Here's how the part is built. I have some questions about the finished solid (model axes, mm). A direction names the side the tool comes from. Give positions to 0.01 mm unless a question says otherwise; leave off trailing zeros. Write each loop counter-clockwise with the first axis right and the second up, starting at its lowest first coordinate (ties: lowest second). Pieces come first, ordered by that corner, then holes. Notation, with made-up numbers: (44.5, 86.25) -> (70.5, 86.25) arc R20 ccw to (70.5, 107.25) -> close; hole circle Ø3 at (73, 4.5). An arc over 180 degrees is marked (long way). Put each result on its own line as item: value. Start each with the question number.
Autodesk Inventor part; units mm, degrees
ref_plane "YZ Plane" through (0, 0, 0) normal (1, 0, 0) x (0, 1, 0)
ref_plane "XZ Plane" through (0, 0, 0) normal (0, 1, 0) x (-1, 0, 0)
ref_plane "XY Plane" through (0, 0, 0) normal (0, 0, 1) x (1, 0, 0)
sketch "Szkic1" plane through (0, 0, 0) normal (1, 0, 0) x (0, 1, 0)
  line L0 (13, 21) -> (0, 21)
  line L1 (0, 21) -> (0, -21)
  line L2 (0, -21) -> (13, -21)
  line L3 (13, -21) -> (13, 21)
  line L4 (0, 0) -> (13, 0) construction
  dimension "d0" = 42
  dimension "d1" = 13
extrude "Wyciągnięcie proste3" add sketch "Szkic1" along normal blind 16
chamfer "Faza1" distance 4 angle 45 2 edges at (8, 0, 21) (8, 0, -21)
sketch "Szkic6" plane through (0, 0, -17) normal (0, -1, 0) x (1, 0, 0)
  line L0 (0, -4) -> (16, -4)
  line L1 (0, 34) -> (0, 0)
  line L2 (16, 34) -> (16, 0)
  point P0 (0, 17)
  point P1 (10, 11)
  dimension "d28" = 15
  dimension "d53" = 6
hole "Otwór2" at (10, 0, -6) direction (0, 1, 0) diameter 3 end through all
sketch "Szkic7" plane through (0, 0, -17) normal (0, -1, 0) x (1, 0, 0)
  line L0 (16, 38) -> (0, 38)
  circle A0 centre (10, 11) radius 1.5
  point P0 (0, 17)
  point P1 (10, 28.5)
  dimension "d37" = 9.5
hole "Otwór3" at (10, 0, 11.5) direction (0, 1, 0) diameter 4 end through all
thread "Gwint2"
sketch "Szkic8" plane through (0, 0, 0) normal (-1, 0, 0) x (0, 0, 1)
  line L0 (21, 13) -> (-17, 13)
  line L1 (-17, 13) -> (-17, 9)
  line L2 (-12, 4) -> (21, 4)
  line L3 (21, 4) -> (21, 13)
  line L4 (17, 0) -> (-17, 0)
  line L5 (-21, 4) -> (-21, 13)
  line L6 (-12, 4) -> (-17, 9)
  point P0 (0, 0)
  point P1 (-17, 4)
  dimension "d55" = 4
  dimension "d56" = 4
  dimension "d59" = 5
  dimension "d60" = 5
extrude "Wyciągnięcie proste5" cut sketch "Szkic8" against normal blind 3
sketch "Szkic9" plane through (16, 0, 0) normal (1, 0, 0) x (0, 0, -1)
  line L0 (-17, 0) -> (17, 0)
  line L1 (21, 4) -> (21, 13)
  point P0 (0, 0)
  point P1 (16.5, 4.5)
  dimension "d63" = 4.5
  dimension "d64" = 4.5
hole "Otwór4" at (16, 4.5, -16.5) direction (-1, 0, 0) diameter 3 end through all
thread "Gwint5"
sketch "Szkic10" plane through (16, 0, 0) normal (1, 0, 0) x (0, 0, -1)
  line L0 (21, 13) -> (-21, 13)
  line L1 (21, 13) -> (9, 13)
  line L2 (9, 13) -> (9, 26)
  line L3 (9, 26) -> (21, 26)
  line L4 (21, 26) -> (21, 13)
  point P0 (0, 0)
  dimension "d74" = 12
  dimension "d75" = 13
extrude "Wyciągnięcie proste6" add sketch "Szkic10" against normal up to surface (16 mm away)
sketch "Szkic11" plane through (0, 0, 0) normal (-1, 0, 0) x (0, 0, 1)
  line L0 (-17, 9) -> (-17, 13)
  line L1 (-9, 26) -> (-21, 26)
  line L2 (-17, 13) -> (-9, 13)
  line L3 (-9, 13) -> (-9, 26)
  line L4 (-9, 26) -> (-17, 26)
  line L5 (-17, 26) -> (-17, 13)
  point P0 (0, 0)
extrude "Wyciągnięcie proste7" cut sketch "Szkic11" against normal up to surface (3 mm away)
fillet "Zaokrąglenie2" radius 2 1 edges at (9.5, 13, -9)
sketch "Szkic12" plane through (16, 0, 0) normal (1, 0, 0) x (0, 0, -1)
  circle A0 centre (16.5, 4.5) radius 1.5
  circle A1 centre (16.5, 4.5) radius 2.75
  point P0 (0, 0)
  dimension "d83" = 1.25
extrude "Wyciągnięcie proste8" cut sketch "Szkic12" against normal blind 3
sketch "Szkic13" plane through (16, 0, 0) normal (1, 0, 0) x (0, 0, -1)
  line L0 (7, 13) -> (-21, 13)
  line L1 (21, 4) -> (21, 26)
  line L2 (7, 13) -> (21, 13)
  line L3 (21, 13) -> (21, 26)
  line L4 (21, 26) -> (7, 26)
  line L5 (7, 26) -> (7, 13)
  point P0 (0, 0)
extrude "Wyciągnięcie proste9" cut sketch "Szkic13" against normal blind 7
thread "Gwint7"
sketch "Szkic14" plane through (9, 0, 0) normal (1, 0, 0) x (0, 0, -1)
  line L0 (21, 26) -> (21, 13)
  line L1 (9, 26) -> (21, 26)
  point P0 (0, 0)
  point P1 (13, 21.5)
  dimension "d90" = 8
  dimension "d91" = 4.5
hole "Otwór5" at (9, 21.5, -13) direction (-1, 0, 0) diameter 3 end through all
thread "Gwint8"
properties part number "34_ekstruder2"
1) I want a section at C-C, the plane y = 21.5. Write out the boundary of the cut face in (x, z), and give its area (3 significant figures).
2) I need wall thicknesses on probe 1 along Z at (x, y) = (10, 7.5); probe 2 along Z at (x, y) = (10, 4.5); probe 3 along Z at (x, y) = (4.6, 21.5). Which ranges of each line are inside material? Lowest first, please.
3) Which directions (+Z, -Z, +X, -X, +Y, -Y) give clear straight access to the entire face, cutting with the end or side of a thin tool? Please do faces 5 (the flat face through (1, 18, -17)), 6 (the flat face through (9, 9, 21)), 7 (the flat face through (6, 20, -9)).
4) I want a section at D-D, the plane y = 11.25. Write out the boundary of the cut face in (x, z).
5) Thinking about a two-plate mould opening in Z: for faces 1 (the flat face through (1, 6, -14)), 2 (the cylindrical face through (14.521, 2.827, -14.318)), 3 (the flat face through (13, 3, -18)), 4 (the flat face through (1, 4, 4)), which applies, released by +Z, released by -Z, zero draft, split by the parting line, or undercut?
6) I want a section at B-B, the plane z = -16.5. Write out the boundary of the cut face in (x, y), and give its area (3 significant figures).
7) I want a section at A-A, the plane x = 10. Write out the boundary of the cut face in (y, z).
8) I'm going to push flat-ended pins straight in: pin 1 Ø1.5 at (x, z) = (1.5, 6.5) entering from +Y; pin 2 Ø4 at (y, z) = (18, -16) entering from +X; pin 3 Ø1.8 at (x, y) = (7, 19.5) entering from +Z. Where does each tip first touch, or does it pass through?
Established:
1. outline: (0, -21) -> (9, -21) -> (9, -14.5) -> (3, -14.5) -> (3, -17) -> (0, -17) -> close; (3, -11.5) -> (9, -11.5) -> (9, -9) -> (3, -9) -> close
1. area: 66.0 mm2
2. probe 1: z = -21 to -7.5, -4.5 to 9.5, 13.5 to 21
2. probe 2: z = -21 to -18, -15 to -7.5, -4.5 to 9.5, 13.5 to 21
2. probe 3: z = -21 to -14.5, -11.5 to -9
3. face 5: +Z, -X, +Y
3. face 6: +Z, +X, -X, +Y, -Y
3. face 7: +Z, +X, -X, +Y
4. outline: (0, -21) -> (16, -21) -> (16, 21) -> (3, 21) -> (3, -17) -> (0, -17) -> close; hole circle Ø4 at (10, 11.5); hole circle Ø3 at (10, -6)
5. face 1: released by +Z
5. face 2: undercut
5. face 3: undercut
5. face 4: zero draft
6. outline: (0, 0) -> (16, 0) -> (16, 1.75) -> (13, 1.75) -> (13, 3) -> (0, 3) -> close; (0, 6) -> (13, 6) -> (13, 7.25) -> (16, 7.25) -> (16, 13) -> (9, 13) -> (9, 26) -> (3, 26) -> (3, 8.5) -> (0, 8.5) -> close
6. area: 217 mm2
7. outline: (0, -17) -> (4, -21) -> (13, -21) -> (13, -7.5) -> (0, -7.5) -> close; (0, -4.5) -> (13, -4.5) -> (13, 9.5) -> (0, 9.5) -> close; (0, 13.5) -> (13, 13.5) -> (13, 21) -> (4, 21) -> (0, 17) -> close; hole circle Ø3 at (4.5, -16.5)
8. pin 1: stops at y = 4
8. pin 2: stops at x = 9
8. pin 3: stops at z = -9
